Geometry: final body of the model. Coordinates: model frame, mm. Face numbers are marked on the shaded views. Give positions to 0.01 mm unless a question says otherwise; leave off trailing zeros. Write each loop counter-clockwise with the first axis right and the second up, starting at its lowest first coordinate (ties: lowest second). Pieces come first, ordered by that corner, then holes. Notation, with made-up numbers: M -21.75,52.25 L 20.25,52.25 A23 ccw 20.25,82.25 Z; hole C 47.5,57 d3. An arc over 180 degrees is marked long. Answer as a JSON object with one key per item and string values.
from build123d import *

# Parameters (mm, degrees)
F0_W        = 381
F0_H        = 273.05
F1_DEPTH    = 38.1
F3_DEPTH    = 273.051
F4_T1_DEPTH = 288.7629933337
F5_R        = 25.4
F6_R        = 6.35


# Not quite as in the source:
# - a fillet or chamfer that OpenCascade refuses, or shapes differently, is made with other operations: its cross-section is extruded or revolved along the edge and cut away or added


with BuildPart() as f1:
    # F0 (on Top) → F1 (new body)
    with BuildSketch(Plane.XY):
        Rectangle(F0_W, F0_H)
    extrude(amount=F1_DEPTH)

    # F2 (on face) → F3 (cut, through all)
    with BuildSketch(Plane.XZ.offset(136.525)):
        with BuildLine():
            Line((152.4, 38.1), (-152.4, 38.1))
            ThreePointArc((-152.4, 38.1), (0, 31.75), (152.4, 38.1))
        make_face()
    extrude(amount=-F3_DEPTH, mode=Mode.SUBTRACT)

    # F4: fillet of radius 76.2 on 2 edges, made by hand

    # F4_s2 → F4_t1 (cut)
    with BuildSketch(Plane.XZ.offset(-144.3814966668)):
        with BuildLine():
            ThreePointArc((155.5425986667, 38.1), (152.4343358341, 38.0365792649), (149.3312469729, 37.846422629))
            ThreePointArc((149.3312469729, 37.846422629), (150.8656767636, 37.9725665634), (152.4, 38.1))
            Line((152.4, 38.1), (155.5425986667, 38.1))
        make_face()
        with BuildLine():
            ThreePointArc((-149.3312469729, 37.846422629), (-152.4343358341, 38.0365792649), (-155.5425986667, 38.1))
            Line((-155.5425986667, 38.1), (-152.4, 38.1))
            ThreePointArc((-152.4, 38.1), (-150.8656767636, 37.9725665634), (-149.3312469729, 37.846422629))
        make_face()
    extrude(amount=F4_T1_DEPTH, mode=Mode.SUBTRACT)

    # F5
    f5_edges = [f1.edges().sort_by_distance(p)[0] for p in [
        (-190.5, -136.525, 19.05),
        (190.5, -136.525, 19.05),
        (190.5, 136.525, 19.05),
        (-190.5, 136.525, 19.05),
    ]]
    fillet(f5_edges, radius=F5_R)

    # F6
    f6_edges = [f1.edges().sort_by_distance(p)[0] for p in [
        (160.321299, 136.525, 38.1),
    ]]
    fillet(f6_edges, radius=F6_R)


solid = f1.part
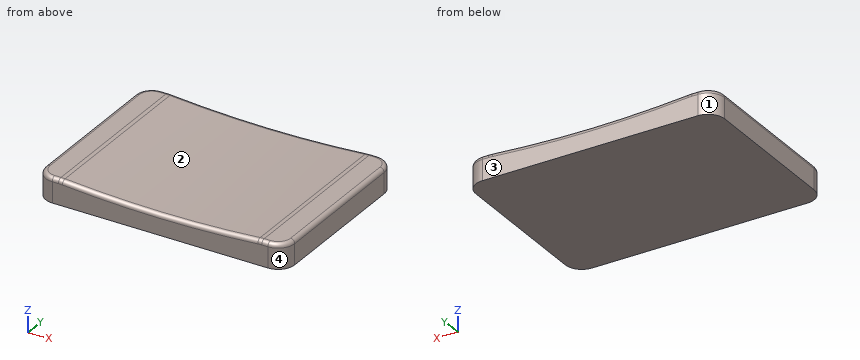
1) Cut plane A-A on y = 16. Return loops of the section in (x, z) (3 decimals).
Geometry check:
{"outline": "M -190.5,0 L 190.5,0 L 190.5,31.75 A6.35 ccw 184.15,38.1 L 155.543,38.1 A76.2 ccw 149.331,37.846 A1831.975 cw -149.331,37.846 A76.2 ccw -155.543,38.1 L -184.15,38.1 A6.35 ccw -190.5,31.75 Z"}
2) Cut plane B-B on x = 0. Return loops of the section in (y, z) (3 decimals), and give its area (3 significant figures).
Geometry check:
{"outline": "M -136.525,0 L 136.525,0 L 136.525,25.4 A6.35 ccw 130.175,31.75 L -130.175,31.75 A6.35 ccw -136.525,25.4 Z", "area": "8,650 mm2"}
3) Contact query for flat-ended pins moving along their axis: P1, Ø3, axis at x = 123.5, y = 24, coming from the +Z side; P2, Ø6, axis at x = 147, y = -90, coming from the +Z side. Output: stop coordinate, or through.
Geometry check:
{"P1": "stops at z = 36.02", "P2": "stops at z = 37.9"}
4) Pull-direction query (X, two-part tool) for the marked faces 1, 2, 3 and 4; classes: pulls with the +X half, pulls with the -X half, needs draft (parallel to the pull), parting line crosses it, or undercut.
Geometry check:
{"face 1": "pulls with the -X half", "face 2": "undercut", "face 3": "needs draft", "face 4": "pulls with the +X half"}
5) Line query: line 1 (Z direction, x = 148.5, y = -70); line 2 (Z direction, x = 150, y = 120); line 3 (Y direction, x = -166, z = 7). Output: solid intervals per line, ascending. Write a range as from..to.
Geometry check:
{"line 1": "z = 0..37.78", "line 2": "z = 0..37.9", "line 3": "y = -136.51..136.51"}
